from build123d import *

# Parameters (mm, degrees)
SKETCH1_W           = 12.8016
SKETCH1_H           = 6.5024
SKETCH1_R           = 1.1684
BOSS_EXTRUDE1_DEPTH = 5.7912
SKETCH2_W           = 1.016
SKETCH2_H           = 3.556
BOSS_EXTRUDE2_DEPTH = 1.27
CUT_EXTRUDE1_DEPTH  = 4.318
BOSS_EXTRUDE6_DEPTH = 5.7912
CUT_EXTRUDE2_DEPTH  = 0.3175
SKETCH7_W           = 0.9525
SKETCH7_H           = 0.635
BOSS_EXTRUDE7_DEPTH = 3.81


with BuildPart() as part:
    # Sketch1 → Boss-Extrude1 (new body)
    with BuildSketch(Plane(origin=(0, 0, 0), x_dir=(1, 0, 0), z_dir=(0, 1, 0))):
        Rectangle(SKETCH1_W, SKETCH1_H)
        with Locations(Location((3.3909, -1.5748, 0), (0, 0, 270))):
            Circle(SKETCH1_R, mode=Mode.SUBTRACT)
        with Locations(Location((-3.3909, -1.5748, 0), (0, 0, 90))):
            Circle(SKETCH1_R, mode=Mode.SUBTRACT)
    extrude(amount=BOSS_EXTRUDE1_DEPTH)

    # Sketch2 → Boss-Extrude2 (add)
    with BuildSketch(Plane(origin=(0, 0, -3.2512), x_dir=(-1, 0, 0), z_dir=(0, 0, -1))):
        with Locations((1.9558, 2.8956)):
            Rectangle(SKETCH2_W, SKETCH2_H)
    extrude(amount=BOSS_EXTRUDE2_DEPTH)

    # Sketch3 → Cut-Extrude1 (cut)
    with BuildSketch(Plane.XZ.offset(-1.1176)):
        with BuildLine():
            Line((-1.4478, -3.2512), (-1.4478, -4.5212))
            Line((-1.4478, -4.5212), (-2.4638, -4.5212))
            Line((-2.4638, -4.5212), (-2.4638, -3.2512))
            ThreePointArc((-2.4638, -3.2512), (-1.9558, -3.7592), (-1.4478, -3.2512))
        make_face()
    extrude(amount=-CUT_EXTRUDE1_DEPTH, mode=Mode.SUBTRACT)

    # Sketch4 → Boss-Extrude6 (add)
    with BuildSketch(Plane(origin=(0, 5.7912, 0), x_dir=(1, 0, 0), z_dir=(0, 1, 0))):
        Polygon((-3.673412994, 3.2512), (-4.744089172, 3.2512), (7.092310828, 6.926499891), (7.092310828, 6.594046101), align=None)
    extrude(amount=-BOSS_EXTRUDE6_DEPTH)

    # Sketch6 → Cut-Extrude2 (cut)
    with BuildSketch(Plane(origin=(-1.337930501, 0, -4.30884038), x_dir=(-0.9550199444571864, 0, 0.29654157497557215), z_dir=(-0.29654157497557215, 0, -0.9550199444571864))):
        Polygon((3.566583809, 0.512911728), (-8.82729348, 1.368515991), (-8.82729348, 0), (3.566583809, 0), align=None)
        with BuildLine():
            Line((3.566583809, 1.689384201), (-0.891541508, 2.163353626))
            ThreePointArc((-0.891541508, 2.163353626), (-1.550065164, 2.8956), (-0.891541508, 3.627846374))
            Line((-0.891541508, 3.627846374), (3.566583809, 4.101815799))
            Line((3.566583809, 4.101815799), (3.566583809, 1.689384201))
        make_face()
        Polygon((3.566583809, 5.278288272), (3.566583809, 5.7912), (-8.82729348, 5.7912), (-8.82729348, 4.422684009), align=None)
    extrude(amount=-CUT_EXTRUDE2_DEPTH, mode=Mode.SUBTRACT)

    # Sketch7 → Boss-Extrude7 (add)
    with BuildSketch(Plane.XY.offset(3.2512)):
        with Locations((-5.1308, 2.8956)):
            Rectangle(SKETCH7_W, SKETCH7_H)
        with Locations((0, 2.8956)):
            Rectangle(SKETCH7_W, SKETCH7_H)
        with Locations((5.1308, 2.8956)):
            Rectangle(SKETCH7_W, SKETCH7_H)
    extrude(amount=BOSS_EXTRUDE7_DEPTH)


solid = part.part
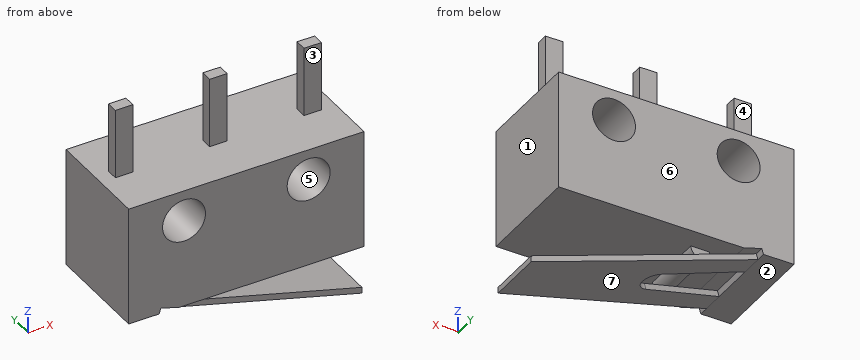
Source: CAD feature listing. Evaluate the final solid. Frame: model axes, mm. Face numbers are marked on the shaded views. A direction names the side the tool comes from. Coordinates: 2 decimals unless noted, no trailing zeros. Loops run counter-clockwise (first coordinate to the right, second up) from the corner with the lowest first, then second, coordinate; pieces in that order, holes last. Notation, with made-up numbers: (5.25, 45) - (47.25, 45) arc R12 cw to (47.25, 64) - close; hole circle Ø9 at (10.5, -21.5). An arc over 180 degrees is marked (long way). Return JSON: item names as keys, results as strings.
Q1. Section D-D, the plane x = -2.75. Return loops of the section in (y, z), plus the area to 3 significant figures.
Results:
{"outline": "(0, -3.25) - (5.79, -3.25) - (5.79, 0.6) - (0, 0.6) - close; (0, 2.55) - (5.79, 2.55) - (5.79, 3.25) - (0, 3.25) - close; (0.65, -3.54) - (0.66, -3.87) - (1.91, -3.87) - (1.9, -3.54) - close; (3.88, -3.87) - (5.13, -3.87) - (5.14, -3.54) - (3.89, -3.54) - close", "area": "27.2 mm2"}
Q2. Access query for the marked faces 1, 2, 3 and 4. Directions: +Z, -Z, +X, -X, +Y, -Y. A direction counts if a zero-diameter tool reaches every point of the face in a straight line with its end or side. Return the directions, or none.
Results:
{"face 1": "+Z, +X, +Y, -Y", "face 2": "-Z, -X, +Y, -Y", "face 3": "+Z, +X, -X, -Y", "face 4": "+Z, +X, -X, +Y"}
Q3. Section B-B, the plane x = 1. Return loops of the section in (y, z), plus the area to 3 significant figures.
Results:
{"outline": "(0, -3.25) - (5.79, -3.25) - (5.79, 3.25) - (0, 3.25) - close; (0.92, -4.7) - (0.93, -5.03) - (4.86, -5.03) - (4.87, -4.7) - close", "area": "39.0 mm2"}
Q4. Section A-A, the plane y = 2.4. Return loops of the section in (x, z).
Results:
{"outline": "(-6.4, -3.25) - (-4.74, -3.25) - (-4.65, -2.95) - (-3.67, -3.25) - (-2.46, -3.25) arc R0.51 ccw to (-1.45, -3.25) - (6.4, -3.25) - (6.4, 3.25) - (-6.4, 3.25) - close; (-0.04, -4.71) - (7.09, -6.93) - (7.09, -6.59) - (0.05, -4.41) - close; hole circle Ø2.34 at (-3.39, 1.57); hole circle Ø2.34 at (3.39, 1.57)"}
Q5. Section C-C, the plane z = 4.5. Return loops of the section in (x, y).
Results:
{"outline": "(-5.61, 2.58) - (-4.65, 2.58) - (-4.65, 3.21) - (-5.61, 3.21) - close; (-0.48, 2.58) - (0.48, 2.58) - (0.48, 3.21) - (-0.48, 3.21) - close; (4.65, 2.58) - (5.61, 2.58) - (5.61, 3.21) - (4.65, 3.21) - close"}
Q6. Material intervals for line 1 along X through (y, z) = (1.45, 2.5); line 2 along Z through (x, y) = (3.75, 4.1); line 3 along Z through (x, y) = (2.5, 2.8), sorted ascending.
Results:
{"line 1": "-6.4 to -4.1, -2.68 to 2.68, 4.1 to 6.4", "line 2": "-5.89 to -5.56, -3.25 to 0.46, 2.69 to 3.25", "line 3": "-5.5 to -5.17, -3.25 to 0.82, 2.33 to 3.25"}
Q7. Contact query for flat-ended pins moving along their axis: P1, Ø0.5, axis at y = 3, z = 5.5, coming from the +X side; P2, Ø0.7, axis at y = 3, z = 5, coming from the -X side; P3, Ø2, axis at x = -3, y = 2, coming from the -Z side. Output: stop coordinate, or through.
Results:
{"P1": "x = 5.61", "P2": "x = -5.61", "P3": "z = -4.1"}
Q8. Mould query, pull axis Z, two halves, no side actions, for the marked faces 5, 6 and 7. Classes: released by +Z, released by -Z, zero draft, split by the parting line, or undercut.
Results:
{"face 5": "undercut", "face 6": "zero draft", "face 7": "released by -Z"}
